from build123d import *

# Parameters (mm, degrees)
CROQUIS1_R              = 3.5
CROQUIS1_W              = 30
CROQUIS1_H              = 3
SALIENTE_EXTRUIR1_DEPTH = 3


with BuildPart() as part:
    # Croquis1 → Saliente-Extruir1 (new body)
    with BuildSketch(Plane.XY):
        Polygon((-190, -67.5), (-97.5, -67.5), (-97.5, -70.5), (-67.5, -70.5), (-67.5, -67.5), (-15, -67.5), (-15, -70.5), (15, -70.5), (15, -67.5), (67.5, -67.5), (67.5, -70.5), (97.5, -70.5), (97.5, -67.5), (190, -67.5), (190, 67.5), (-190, 67.5), align=None)
        with Locations((-170, -37.5)):
            Circle(CROQUIS1_R, mode=Mode.SUBTRACT)
        with Locations((170, -37.5)):
            Circle(CROQUIS1_R, mode=Mode.SUBTRACT)
        with Locations((82.5, -29)):
            Rectangle(CROQUIS1_W, CROQUIS1_H, mode=Mode.SUBTRACT)
        with Locations((0, -29)):
            Rectangle(CROQUIS1_W, CROQUIS1_H, mode=Mode.SUBTRACT)
        with Locations((-82.5, -29)):
            Rectangle(CROQUIS1_W, CROQUIS1_H, mode=Mode.SUBTRACT)
    extrude(amount=SALIENTE_EXTRUIR1_DEPTH)


solid = part.part
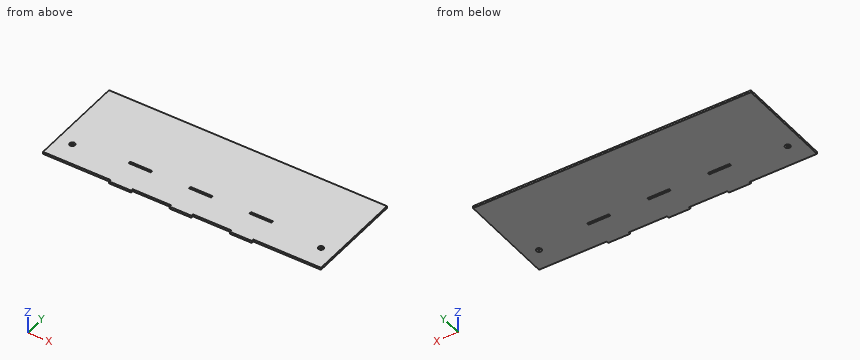
Read the model definition and answer for the solid it produces. Units are mm, in the model's axes. Round coordinates to 2 decimals unless told otherwise and drop trailing zeros. Write each loop counter-clockwise with the first axis right and the second up, starting at its lowest first coordinate (ties: lowest second). Pieces come first, ordered by that corner, then holes. Notation, with made-up numbers: (-16.75, 27.25) - (-1.75, 27.25) arc R26 cw to (-1.75, 60.25) - close; hole circle Ø7 at (-15, -26). An arc over 180 degrees is marked (long way). One line per question, with ' | ' between items. Start each with the question number.
1. Each of these flat-tipped pins is pushed along its axis until it touches: pin 1 (1 mm diameter, centred on x = -16.5, y = 15, fed in from -Z); pin 2 (1.5 mm diameter, centred on y = -69, z = 1, fed in from -X); pin 3 (1.5 mm diameter, centred on y = -68.5, z = 1.5, fed in from +X); pin 4 (0.9 mm diameter, centred on x = 47, z = 1, fed in from -Y). Where does it stop, or does it pass through?
2. Section C-C (y = -37.5) is taken. Determine the outline of the cut face in (x, z).
3. Section D-D (x = 91.5) is taken. Determine the outline of the cut face in (y, z), and give its area (3 significant figures).
4. Section B-B (z = 1) is taken. Give the number of separate pieces and of enclosed holes in the cut face, and give its area (3 significant figures).
5. Find the intervals of material crossed by probe 1 along Y at (x, z) = (-170, 2.2); probe 2 along Y at (x, z) = (-93.5, 0.2); probe 3 along X at (y, z) = (-35.5, 0.25), in increasing order. Write a range as [from, to].
6. Section A-A (x = 170) is taken. Determine the outline of the cut face in (y, z), and give its area (3 significant figures).
Filled in:
1) pin 1: z = 0 | pin 2: x = -97.5 | pin 3: x = 97.5 | pin 4: y = -67.5
2) outline: (-190, 0) - (-173.5, 0) - (-173.5, 3) - (-190, 3) - close; (-166.5, 0) - (166.5, 0) - (166.5, 3) - (-166.5, 3) - close; (173.5, 0) - (190, 0) - (190, 3) - (173.5, 3) - close
3) outline: (-70.5, 0) - (-30.5, 0) - (-30.5, 3) - (-70.5, 3) - close; (-27.5, 0) - (67.5, 0) - (67.5, 3) - (-27.5, 3) - close | area: 405 mm²
4) separate pieces: 1 | enclosed holes: 5 | area: 51,200 mm²
5) probe 1: [-67.5, -41], [-34, 67.5] | probe 2: [-70.5, -30.5], [-27.5, 67.5] | probe 3: [-190, -172.87], [-167.13, 167.13], [172.87, 190]
6) outline: (-67.5, 0) - (-41, 0) - (-41, 3) - (-67.5, 3) - close; (-34, 0) - (67.5, 0) - (67.5, 3) - (-34, 3) - close | area: 384 mm²
